Read the model definition and answer for the solid it produces. Units are mm, in the model's axes. Give positions to 0.01 mm unless a question says otherwise; leave off trailing zeros. Write each loop counter-clockwise with the first axis right and the second up, starting at its lowest first coordinate (ties: lowest second). Pieces come first, ordered by that corner, then holes. Notation, with made-up numbers: (-14, 55) -> (33, 55) arc R31 ccw to (33, 85) -> close; hole circle Ø2 at (-34.75, 88). An arc over 180 degrees is marked (long way). Write item = value, one per line.
from build123d import *

# Parameters (mm, degrees)
SKETCH1_R        = 1.85915493
SKETCH1_R_2      = 1.983111479
EXTRUSION1_DEPTH = 1.6
FILLET1_R        = 1
FILLET2_R        = 4
FILLET3_R        = 3
FILLET4_R        = 3
FILLET5_R        = 2
FILLET6_R        = 2
FILLET7_R        = 3
FILLET8_R        = 3
FILLET9_R        = 2
FILLET10_R       = 2
FILLET11_R       = 3


with BuildPart() as part:
    # Sketch1 → Extrusion1 (new body)
    with BuildSketch(Plane(origin=(0, 0, 0), x_dir=(-1, 0, 0), z_dir=(0, 1, 0))):
        Polygon((74.087520418, 321.088295015), (70.369210559, 327.285477572), (45.580478165, 327.285477572), (45.580478165, 312.412238135), (23.246043749, 290.934342561), (26.682507041, 287.360833055), (12.735407819, 253.538985229), (9.017097883, 253.538985229), (9.017097883, 226.891111382), (9.017097883, 200.243237534), (12.735407819, 200.243237534), (26.682507041, 166.421389708), (23.246043749, 162.847880202), (45.580478165, 141.369984628), (45.580478165, 126.496745191), (70.369210559, 126.496745191), (74.087520418, 132.693927748), (97.636816193, 132.693927748), (121.186111968, 132.693927748), (124.904421827, 126.496745191), (149.693154221, 126.496745191), (149.693154221, 141.369984628), (172.027588636, 162.847880202), (168.591125345, 166.421389708), (182.538224567, 200.243237534), (186.256534503, 200.243237534), (186.256534503, 226.891111382), (186.256534503, 253.538985229), (182.538224567, 253.538985229), (168.591125345, 287.360833055), (172.027588636, 290.934342561), (149.693154221, 312.412238135), (149.693154221, 327.285477572), (124.904421827, 327.285477572), (121.186111968, 321.088295015), (97.636816193, 321.088295015), align=None)
        with Locations((49.266182018, 151.62213525)):
            Circle(SKETCH1_R, mode=Mode.SUBTRACT)
        with Locations((51.777661187, 316.130534525)):
            Circle(SKETCH1_R, mode=Mode.SUBTRACT)
        with Locations((49.266182018, 302.160087513)):
            Circle(SKETCH1_R, mode=Mode.SUBTRACT)
        with Locations((143.495971199, 137.651688238)):
            Circle(SKETCH1_R, mode=Mode.SUBTRACT)
        with Locations((146.007450368, 151.62213525)):
            Circle(SKETCH1_R, mode=Mode.SUBTRACT)
        with Locations((143.495971199, 316.130534525)):
            Circle(SKETCH1_R, mode=Mode.SUBTRACT)
        with Locations((146.007450368, 302.160087513)):
            Circle(SKETCH1_R, mode=Mode.SUBTRACT)
        with Locations((51.777661187, 137.651688238)):
            Circle(SKETCH1_R, mode=Mode.SUBTRACT)
        with Locations((67.636816193, 196.891111382)):
            Circle(SKETCH1_R_2, mode=Mode.SUBTRACT)
        with Locations((67.636816193, 256.891111382)):
            Circle(SKETCH1_R_2, mode=Mode.SUBTRACT)
        with Locations((42.888078851, 158.000238416)):
            Circle(SKETCH1_R, mode=Mode.SUBTRACT)
        with Locations((152.385553534, 295.781984347)):
            Circle(SKETCH1_R, mode=Mode.SUBTRACT)
        with Locations((42.888078851, 295.781984347)):
            Circle(SKETCH1_R, mode=Mode.SUBTRACT)
        with Locations((127.636816193, 256.891111382)):
            Circle(SKETCH1_R_2, mode=Mode.SUBTRACT)
        with Locations((152.385553534, 158.000238416)):
            Circle(SKETCH1_R, mode=Mode.SUBTRACT)
        with Locations((127.636816193, 196.891111382)):
            Circle(SKETCH1_R_2, mode=Mode.SUBTRACT)
    extrude(amount=EXTRUSION1_DEPTH)

    # Fillet1
    fillet1_edges = [part.edges().sort_by_distance(p)[0] for p in [
        (-121.186111968, 0.8, 321.088295015),
        (-121.186111968, 0.8, 132.693927748),
        (-74.087520418, 0.8, 132.693927748),
        (-74.087520418, 0.8, 321.088295015),
    ]]
    fillet(fillet1_edges, radius=FILLET1_R)

    # Fillet2
    fillet2_edges = [part.edges().sort_by_distance(p)[0] for p in [
        (-149.693154221, 0.8, 327.285477572),
        (-149.693154221, 0.8, 126.496745191),
        (-45.580478165, 0.8, 126.496745191),
        (-45.580478165, 0.8, 327.285477572),
    ]]
    fillet(fillet2_edges, radius=FILLET2_R)

    # Fillet3
    fillet3_edges = [part.edges().sort_by_distance(p)[0] for p in [
        (-149.693154221, 0.8, 312.412238135),
        (-149.693154221, 0.8, 141.369984628),
        (-45.580478165, 0.8, 141.369984628),
        (-45.580478165, 0.8, 312.412238135),
    ]]
    fillet(fillet3_edges, radius=FILLET3_R)

    # Fillet4
    fillet4_edges = [part.edges().sort_by_distance(p)[0] for p in [
        (-172.027588636, 0.8, 290.934342561),
    ]]
    fillet(fillet4_edges, radius=FILLET4_R)

    # Fillet5
    fillet5_edges = [part.edges().sort_by_distance(p)[0] for p in [
        (-168.591125345, 0.8, 287.360833055),
    ]]
    fillet(fillet5_edges, radius=FILLET5_R)

    # Fillet6
    fillet6_edges = [part.edges().sort_by_distance(p)[0] for p in [
        (-26.682507041, 0.8, 287.360833055),
    ]]
    fillet(fillet6_edges, radius=FILLET6_R)

    # Fillet7
    fillet7_edges = [part.edges().sort_by_distance(p)[0] for p in [
        (-23.246043749, 0.8, 290.934342561),
    ]]
    fillet(fillet7_edges, radius=FILLET7_R)

    # Fillet8
    fillet8_edges = [part.edges().sort_by_distance(p)[0] for p in [
        (-172.027588636, 0.8, 162.847880202),
        (-23.246043749, 0.8, 162.847880202),
    ]]
    fillet(fillet8_edges, radius=FILLET8_R)

    # Fillet9
    fillet9_edges = [part.edges().sort_by_distance(p)[0] for p in [
        (-168.591125345, 0.8, 166.421389708),
        (-26.682507041, 0.8, 166.421389708),
    ]]
    fillet(fillet9_edges, radius=FILLET9_R)

    # Fillet10
    fillet10_edges = [part.edges().sort_by_distance(p)[0] for p in [
        (-182.538224567, 0.8, 253.538985229),
        (-182.538224567, 0.8, 200.243237534),
        (-12.735407819, 0.8, 200.243237534),
        (-12.735407819, 0.8, 253.538985229),
    ]]
    fillet(fillet10_edges, radius=FILLET10_R)

    # Fillet11
    fillet11_edges = [part.edges().sort_by_distance(p)[0] for p in [
        (-186.256534503, 0.8, 200.243237534),
        (-186.256534503, 0.8, 253.538985229),
        (-9.017097883, 0.8, 253.538985229),
        (-9.017097883, 0.8, 200.243237534),
    ]]
    fillet(fillet11_edges, radius=FILLET11_R)


solid = part.part
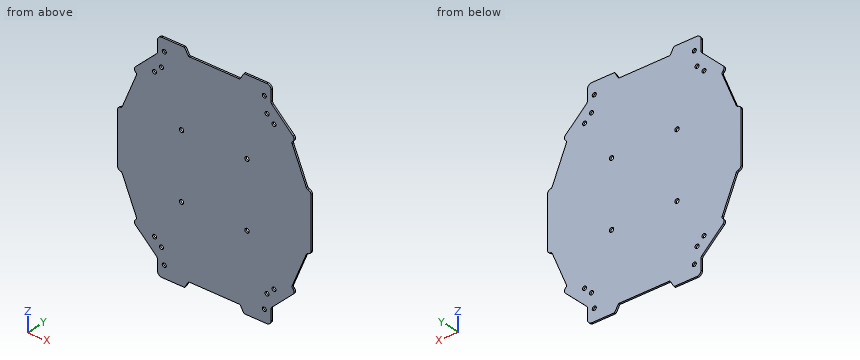
(1) The part is cut by section A-A on x = -106. Determine the outline of the cut face in (y, z).
Checks:
outline = (0, 132.69) -> (1.6, 132.69) -> (1.6, 321.09) -> (0, 321.09) -> close
(2) The part is cut by section B-B on y = 1.3. Count the separate pieces of the cut face and the enclosed holes in it, plus the area to 3 significant figures.
Checks:
separate_pieces = 1
enclosed_holes = 16
area = 28,700 mm²
(3) Consider L1, parallel to X at y = 0.75, z = 316; L2, parallel to X at y = 0.4, z = 158.5; L3, parallel to Z at x = -66, y = 0.25. Determine where each line is inside the solid, lowest interval first.
Checks:
L1 = -149.69 to -145.35, -141.64 to -53.63, -49.92 to -45.58
L2 = -167.51 to -154.18, -150.59 to -44.68, -41.1 to -27.77
L3 = 126.5 to 195.77, 198.01 to 255.77, 258.01 to 327.29
(4) Given P1, Ø0.8, axis at x = -100.5, y = 0.5, coming from the +Z side; P2, Ø3, axis at x = -51.78, z = 316.13, coming from the -Y side; P3, Ø0.8, axis at y = 0.5, z = 134, coming from the +X side, each flat-ended and moving along its own axis, determine where each tip first touches the part or whether it passes through.
Checks:
P1 = 321.09
P2 = through
P3 = -45.58
(5) The part is cut by section C-C on z = 277. Determine the outline of the cut face in (x, y).
Checks:
outline = (-172.86, 0) -> (-22.41, 0) -> (-22.41, 1.6) -> (-172.86, 1.6) -> close
